```python
from build123d import *

# Parameters (mm, degrees)
F2_R     = 38.1
F3_DEPTH = 6.35
F6_R     = 12.7
F6_R_2   = 9.525
F7_DEPTH = 50.8
F9_DEPTH = 25.4


with BuildPart() as f3:
    # F2 (on face) → F3 (new body)
    with BuildSketch(Plane(origin=(0, 0, 0), x_dir=(-1, 0, 0), z_dir=(0, 0.970296, 0.241922))):
        Circle(F2_R)
    extrude(amount=F3_DEPTH)

    # F6 (on face) → F7 (join)
    with BuildSketch(Plane(origin=(0, 0, 0), x_dir=(-1, 0, 0), z_dir=(0, 0.970296, 0.241922))):
        Circle(F6_R)
        Circle(F6_R_2, mode=Mode.SUBTRACT)
    extrude(amount=F7_DEPTH)

    # F8 (on Right) → F9 (cut)
    with BuildSketch(Plane.YZ):
        Polygon((3.551053, -14.242495), (-5.652468, 22.670809), (-19.892405, 18.754688), (-9.609196, -17.931353), align=None)
    extrude(amount=-F9_DEPTH, mode=Mode.SUBTRACT)


solid = f3.part
```
Build history of the part. All positions in model axes, mm. Give positions to 0.01 mm unless a question says otherwise; leave off trailing zeros. Loops run counter-clockwise (first coordinate to the right, second up) from the corner with the lowest first, then second, coordinate; pieces in that order, holes last.
Item 1: Slice it at A-A, the plane x = 1. List the corners of the cut face in (y, z), and give its area (3 significant figures).
Answers follow:
outline: (-9.21, 36.96) - (9.21, -36.96) - (15.38, -35.42) - (9.22, -10.75) - (52.35, 0.01) - (51.58, 3.1) - (8.45, -7.65) - (3.87, 10.73) - (47, 21.48) - (46.23, 24.57) - (3.1, 13.82) - (-3.05, 38.49) - close
area: 767 mm2
Item 2: Slice it at D-D, the plane x = 24. List the corners of the cut face in (y, z), and give its area (3 significant figures).
Answers follow:
outline: (-7.16, 28.71) - (7.16, -28.71) - (13.32, -27.18) - (-1, 30.25) - close
area: 376 mm2
Item 3: Pull direction Y, two halves, no side cores. Call faces 1 (the face through (30.23, 8.65, -21.74)), 2 (the face through (0.53, -0.13, 0.52)), 3 (the face through (0.13, 6.13, 1.67)): released by +Y, released by -Y, zero draft, split by the parting line, or undercut.
Answers follow:
face 1: split by the parting line
face 2: released by -Y
face 3: undercut
Item 4: Slice it at C-C, the plane x = -18. List the corners of the cut face in (y, z), and give its area (3 significant figures).
Answers follow:
outline: (-8.12, 32.58) - (8.12, -32.58) - (14.29, -31.05) - (-1.96, 34.12) - close
area: 426 mm2
Item 5: Flat gauge pins, fed straight in: pin 1 (1 mm diameter, centred on x = -8.5, z = 15.5, fed in from +Y); pin 2 (12 mm diameter, centred on x = 10.5, y = 15, fed in from +Z); pin 3 (5 mm diameter, centred on x = 0, z = 12, fed in from -Y); pin 4 (12 mm diameter, centred on y = 33.5, z = -11.5, fed in from -X). Where does each tip first touch, or does it go through?
Answers follow:
pin 1: stops at y = 48.52
pin 2: stops at z = 16.38
pin 3: stops at y = -3.62
pin 4: passes through
Item 6: Drill centre lines: line 1 (X direction, y = 23, z = 4.5); line 2 (Z direction, x = 2, y = 44.5); line 3 (Y direction, x = 0.5, z = 8). Where is each one in solid material? Low to high.
Answers follow:
line 1: x = -12.64 to -9.45, 9.45 to 12.64
line 2: z = -1.83 to 1.5, 20.69 to 24.02
line 3: y = -1.99 to 4.55
Item 7: Slice it at B-B, the plane y = 13.5. Give the number of separate pieces and of enclosed holes in the cut face, and give its area (3 significant figures).
Answers follow:
separate pieces: 2
enclosed holes: 1
area: 480 mm2
